Job drawing, mm, ordinate dimensions from the low corner. One solid piece. A direction names the side the tool comes from. Give positions to 0.01 mm unless a question says otherwise; leave off trailing zeros. Order: outer loops, then holes, each group sorted by start corner. A loop starts at its lowest first (then second) coordinate and runs counter-clockwise, first axis right, second up. Notation, with made-up numbers: M 13,59.25 L 19,59.25 A21 ccw 19,94.25 Z; hole C -33.5,2 d3. An arc over 180 degrees is marked long. Put each result on its own line as item: value. Start each with the question number.
1) Cut at C-C (z = 30). Write the cut outline in (x, y).
2) Drill centre lines: line 1 (Z direction, x = 34, y = 2.05); line 2 (Y direction, x = 1, z = 30); line 3 (X direction, y = 25, z = 17). Where is each one in solid material? Low to high. Write a range as [from, to].
3) Tool access for the marked faces 1 and 2: list every direction of +Z, -Z, +X, -X, +Y, -Y with a clear straight run to the whole face (end or side of a thin tool).
4) Pin check, flat tips, straight feed: pin 1 (10 mm diameter, centred on x = 14, y = 11, fed in from +Z); pin 2 (5 mm diameter, centred on y = 34.5, z = 12, fed in from +X); pin 3 (6 mm diameter, centred on y = 14, z = 30, fed in from -X); pin 4 (5 mm diameter, centred on x = 34, z = 10, fed in from +Y). Stop position of each tip, or through.
5) Cut at A-A (x = 14). Write the cut outline in (y, z), and give its area (3 significant figures).
6) Cut at D-D (z = 5.5). Write the cut outline in (x, y).
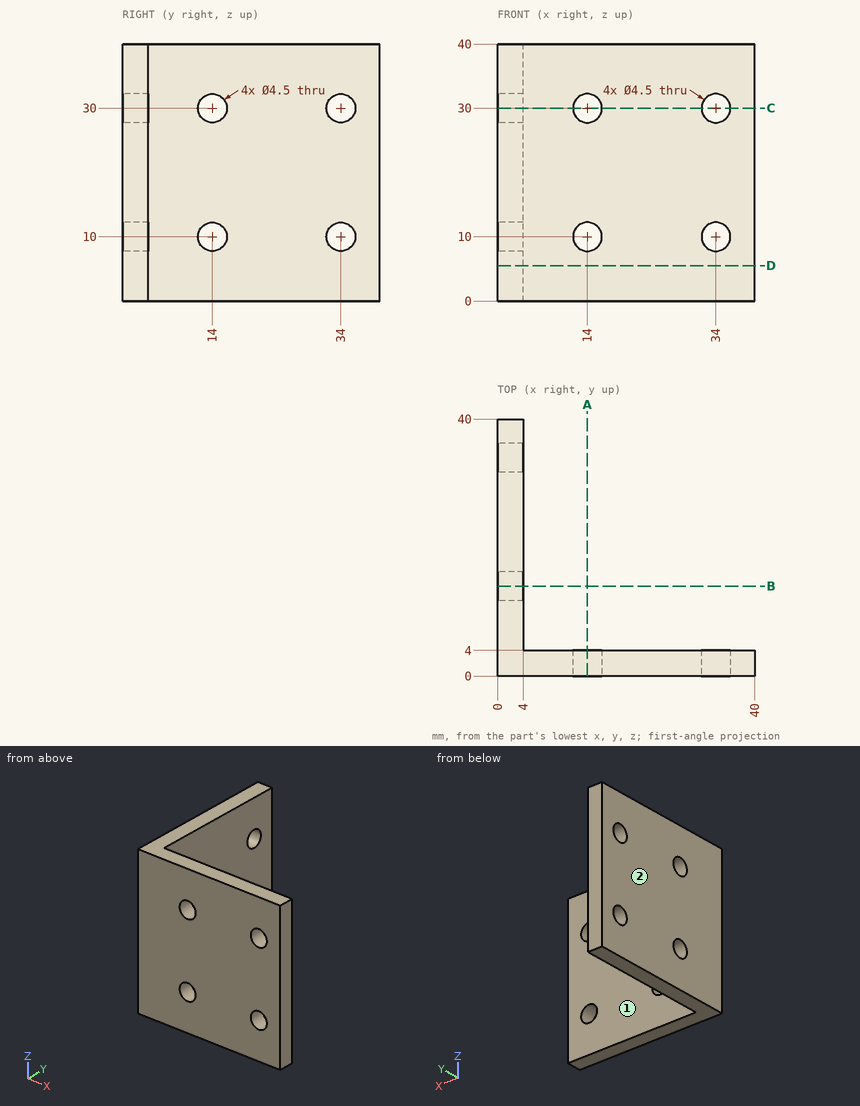
Solution:
1. outline: M 0,0 L 11.75,0 L 11.75,4 L 4,4 L 4,11.75 L 0,11.75 Z; M 0,16.25 L 4,16.25 L 4,31.75 L 0,31.75 Z; M 0,36.25 L 4,36.25 L 4,40 L 0,40 Z; M 16.25,0 L 31.75,0 L 31.75,4 L 16.25,4 Z; M 36.25,0 L 40,0 L 40,4 L 36.25,4 Z
2. line 1: [0, 7.75], [12.25, 27.75], [32.25, 40]
2. line 2: [0, 11.75], [16.25, 31.75], [36.25, 40]
2. line 3: [0, 4]
3. face 1: +Z, -Z, +X, +Y
3. face 2: +Z, -Z, -X, +Y, -Y
4. pin 1: through
4. pin 2: x = 4
4. pin 3: x = 0
4. pin 4: y = 4
5. outline: M 0,0 L 4,0 L 4,7.75 L 0,7.75 Z; M 0,12.25 L 4,12.25 L 4,27.75 L 0,27.75 Z; M 0,32.25 L 4,32.25 L 4,40 L 0,40 Z
5. area: 124 mm²
6. outline: M 0,0 L 40,0 L 40,4 L 4,4 L 4,40 L 0,40 Z
